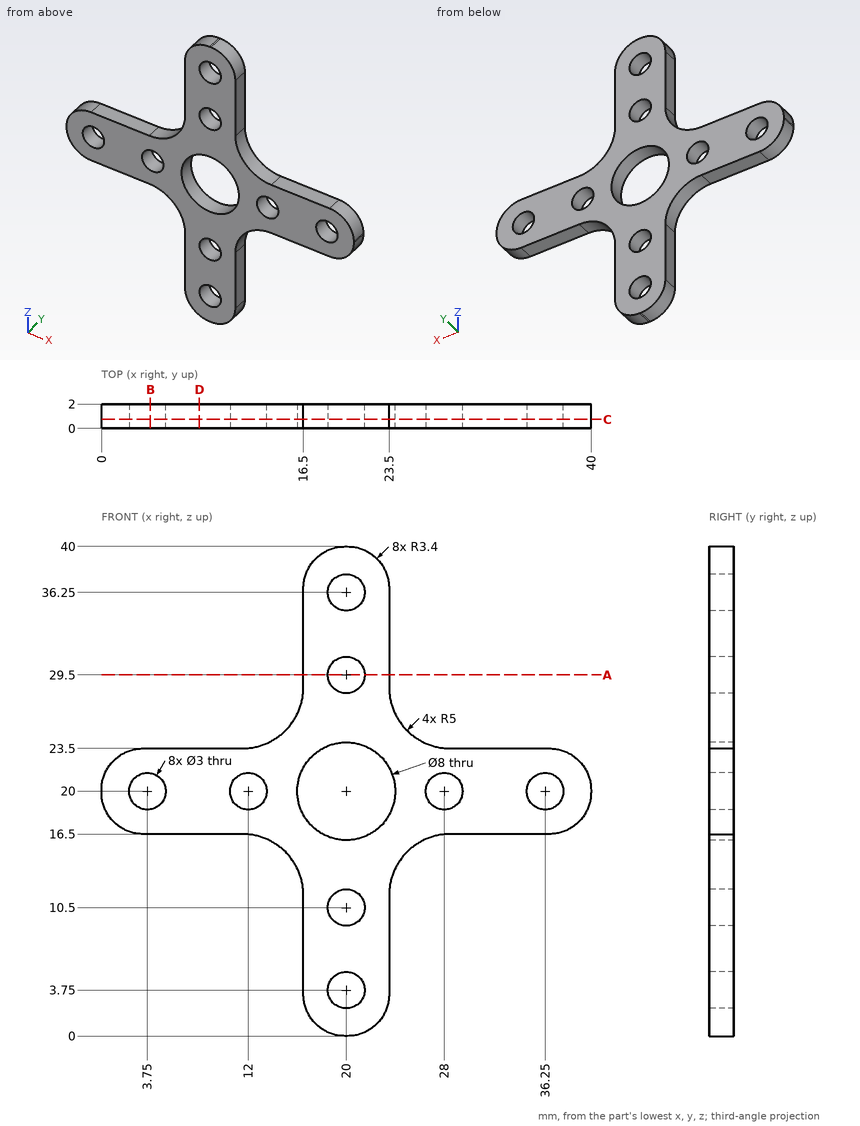
Print and shaded views of the part. All mm, measured from the part's lowest x, y and z. Round coordinates to 2 decimals unless told otherwise and drop trailing zeros. Write each loop counter-clockwise with the first axis right and the second up, starting at its lowest first coordinate (ties: lowest second). Pieces come first, ordered by that corner, then holes. Notation, with made-up numbers: (50.5, 39) -> (101.5, 39) arc R31 cw to (101.5, 77) -> close; hole circle Ø4 at (-25, 17). An arc over 180 degrees is marked (long way). Return JSON: item names as keys, results as strings. Group by question number.
Q1. Saw through at B-B on x = 4. Write the cut outline in (y, z), plus the area to 3 significant figures.
Q2. Probe L1, parallel to X at y = 1.4, z = 20; L2, parallel to X at y = 0.9, z = 3.75; L3, parallel to X at y = 0.5, z = 21. List the from-to ranges inside material, lowest first. Write a range as [from, to].
Q3. Pin check, flat tips, straight feed: pin 1 (0.6 mm diameter, centred on x = 6.5, y = 0.5, fed in from -Z); pin 2 (1 mm diameter, centred on x = 34, y = 0.5, fed in from +Z); pin 3 (0.6 mm diameter, centred on y = 1, z = 31, fed in from -X). Stop position of each tip, or through.
Q4. Saw through at C-C on y = 0.75. State how many separate pieces and enclosed holes the cut face has, plus the area to 3 significant figures.
Q5. Saw through at D-D on x = 8. Write the cut outline in (y, z), plus the area to 3 significant figures.
Q6. Saw through at A-A on z = 29.5. Write the cut outline in (x, y).
Answer:
{
 "1": {"outline": "(0, 16.5) -> (2, 16.5) -> (2, 18.52) -> (0, 18.52) -> close; (0, 21.48) -> (2, 21.48) -> (2, 23.5) -> (0, 23.5) -> close", "area": "8.08 mm2"},
 "2": {"L1": "[0, 2.25], [5.25, 10.5], [13.5, 16], [24, 26.5], [29.5, 34.75], [37.75, 40]", "L2": "[16.5, 18.5], [21.5, 23.5]", "L3": "[0.12, 2.63], [4.87, 10.88], [13.12, 16.13], [23.87, 26.88], [29.12, 35.13], [37.37, 39.88]"},
 "3": {"pin 1": "z = 16.5", "pin 2": "z = 23.5", "pin 3": "x = 16.5"},
 "4": {"separate pieces": "1", "enclosed holes": "9", "area": "406 mm2"},
 "5": {"outline": "(0, 16.5) -> (2, 16.5) -> (2, 23.5) -> (0, 23.5) -> close", "area": "14.0 mm2"},
 "6": {"outline": "(16.5, 0) -> (18.5, 0) -> (18.5, 2) -> (16.5, 2) -> close; (21.5, 0) -> (23.5, 0) -> (23.5, 2) -> (21.5, 2) -> close"}
}
